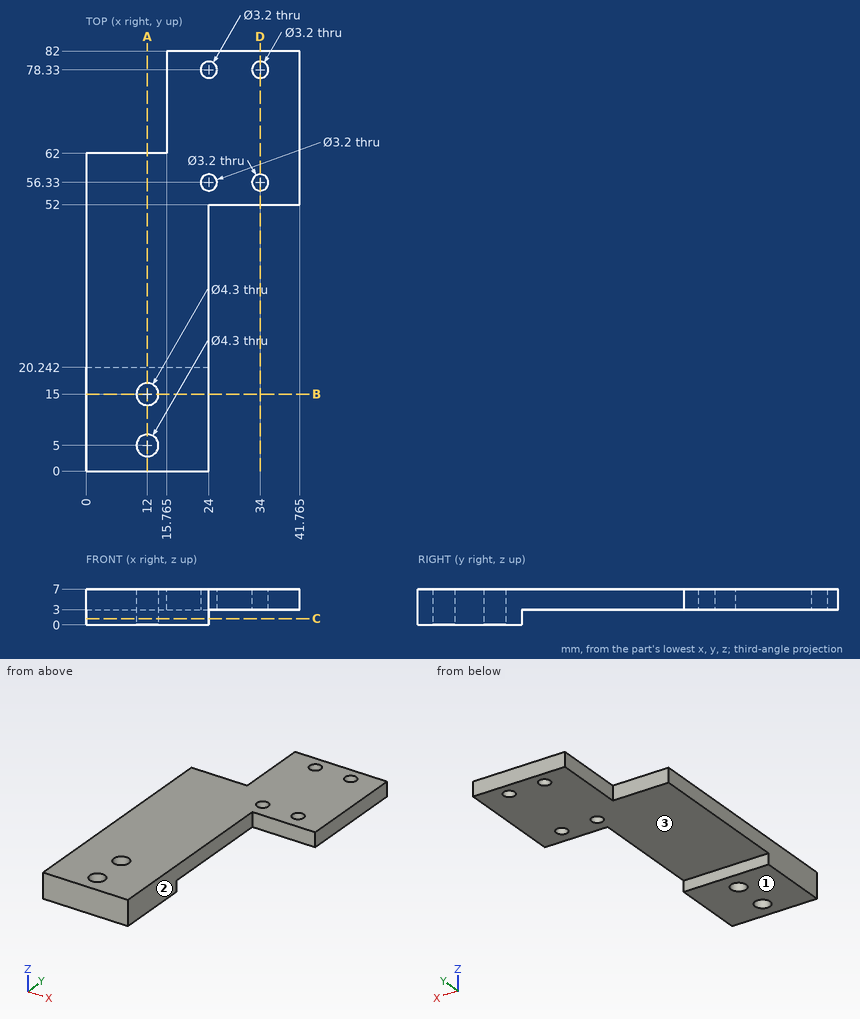
The drawing under review shows one solid part. Ordinate dimensions are in mm from its lowest x, y, z. A direction names the side the tool comes from. Coordinates: 2 decimals unless noted, no trailing zeros. Write each loop counter-clockwise with the first axis right and the second up, starting at its lowest first coordinate (ties: lowest second). Pieces come first, ordered by that corner, then holes. Notation, with made-up numbers: (38.5, -27) -> (71.5, -27) arc R25 ccw to (71.5, 7) -> close; hole circle Ø8 at (25.5, 81). An arc over 180 degrees is marked (long way). One line per item, written item: value. Start each with the question number.
Q1. Add section B-B, the plane y = 15. Give the boundary of the cut face in (x, z).
Q2. To check wall thickness, follow probe 1 along Y at (x, z) = (12, 1.75); probe 2 along Y at (x, z) = (12, 4.25); probe 3 along Z at (x, y) = (15.5, 49.5). State the ranges of each line that lie inside material, in increasing order.
Q3. Add section A-A, the plane x = 12. Give the boundary of the cut face in (y, z).
Q4. Add section C-C, the plane z = 1.25. Give the boundary of the cut face in (x, y).
Q5. Add section D-D, the plane x = 34. Give the boundary of the cut face in (y, z).
Q6. Clearance check with flat-ended pins moving along their axes: P1, Ø3, axis at x = 4.5, z = 4, coming from the +Y side; P2, Ø12.5, axis at x = 14, y = 48.5, coming from the -Z side; P3, Ø3, axis at x = 32.5, z = 5.5, coming from the -Y side. State where each tip first meets the part, or that it passes through.
Q7. For the marked faces 1, 2 and 3, list the 3-axis set-ups (+Z, -Z, +X, -X, +Y, -Y) from which the entire face can be reached by the end or side of a thin tool; tool diameter is ignored.
Response:
1. outline: (0, 0) -> (9.85, 0) -> (9.85, 7) -> (0, 7) -> close; (14.15, 0) -> (24, 0) -> (24, 7) -> (14.15, 7) -> close
2. probe 1: 0 to 2.85, 7.15 to 12.85, 17.15 to 20.24
2. probe 2: 0 to 2.85, 7.15 to 12.85, 17.15 to 62
2. probe 3: 3 to 7
3. outline: (0, 0) -> (2.85, 0) -> (2.85, 7) -> (0, 7) -> close; (7.15, 0) -> (12.85, 0) -> (12.85, 7) -> (7.15, 7) -> close; (17.15, 0) -> (20.24, 0) -> (20.24, 3) -> (62, 3) -> (62, 7) -> (17.15, 7) -> close
4. outline: (0, 0) -> (24, 0) -> (24, 20.24) -> (0, 20.24) -> close; hole circle Ø4.3 at (12, 5); hole circle Ø4.3 at (12, 15)
5. outline: (52, 3) -> (54.73, 3) -> (54.73, 7) -> (52, 7) -> close; (57.93, 3) -> (76.73, 3) -> (76.73, 7) -> (57.93, 7) -> close; (79.93, 3) -> (82, 3) -> (82, 7) -> (79.93, 7) -> close
6. P1: y = 62
6. P2: z = 3
6. P3: y = 52
7. face 1: -Z, +X, -X, +Y, -Y
7. face 2: +Z, -Z, +X, -Y
7. face 3: -Z, +X, -X, +Y
